Here's how the part is built. I have some questions about the finished solid (model axes, mm). Round coordinates to 2 decimals unless told otherwise and drop trailing zeros. Loops run counter-clockwise (first coordinate to the right, second up) from the corner with the lowest first, then second, coordinate; pieces in that order, holes last. Notation, with made-up numbers: (-18, -22.5) - (26, -22.5) arc R28 cw to (26, -2.5) - close; hole circle Ø4 at (12.5, 31.5). An arc over 180 degrees is marked (long way). Return JSON: item names as keys, results as strings. Group by question number.
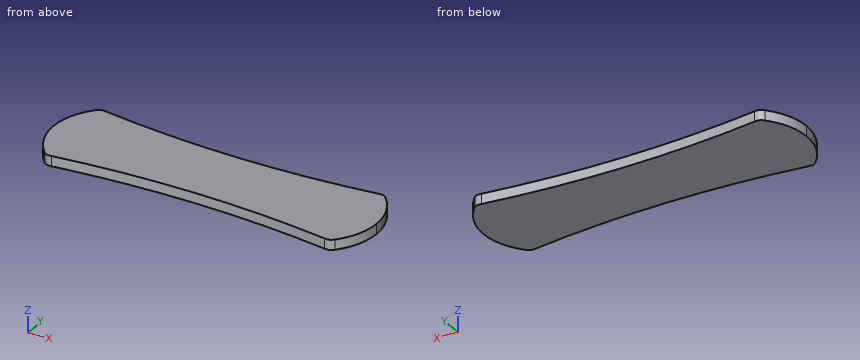
```python
from build123d import *

# Parameters (mm, degrees)
F1_DEPTH    = 25.4
F2_T1_DEPTH = 93.9988541888


# Not quite as in the source:
# - a fillet or chamfer that OpenCascade refuses, or shapes differently, is made with other operations: its cross-section is extruded or revolved along the edge and cut away or added


with BuildPart() as f1:
    # F0 (on Top) → F1 (new body)
    with BuildSketch(Plane.XY):
        with BuildLine():
            ThreePointArc((50.8, 558.8), (13.2719441568, 507.0402470414), (0, 444.5))
            ThreePointArc((0, 444.5), (13.2719441568, 381.9597529586), (50.8, 330.2))
            Line((50.8, 330.2), (50.8, 558.8))
        make_face()
        with BuildLine():
            ThreePointArc((277.2968022896, 536.7332159534), (163.7973759268, 545.1900472484), (50.8, 558.8))
            Line((50.8, 558.8), (50.8, 330.2))
            ThreePointArc((50.8, 330.2), (163.7973759268, 343.8099527516), (277.2968022896, 352.2667840466))
            ThreePointArc((277.2968022896, 352.2667840466), (300.1043048901, 395.8992851393), (307.975, 444.5))
            ThreePointArc((307.975, 444.5), (300.1043048901, 493.1007148607), (277.2968022896, 536.7332159534))
        make_face()
        with BuildLine():
            Line((762, 330.2), (762, 558.8))
            ThreePointArc((762, 558.8), (649.0026240732, 545.1900472484), (535.5031977104, 536.7332159534))
            ThreePointArc((535.5031977104, 536.7332159534), (504.825, 444.5), (535.5031977104, 352.2667840466))
            ThreePointArc((535.5031977104, 352.2667840466), (649.0026240732, 343.8099527516), (762, 330.2))
        make_face()
        with BuildLine():
            ThreePointArc((812.8, 444.5), (799.5280558432, 507.0402470414), (762, 558.8))
            Line((762, 558.8), (762, 330.2))
            ThreePointArc((762, 330.2), (799.5280558432, 381.9597529586), (812.8, 444.5))
        make_face()
        with BuildLine():
            ThreePointArc((535.5031977104, 536.7332159534), (406.4, 533.4), (277.2968022896, 536.7332159534))
            ThreePointArc((277.2968022896, 536.7332159534), (300.1043048901, 493.1007148607), (307.975, 444.5))
            ThreePointArc((307.975, 444.5), (300.1043048901, 395.8992851393), (277.2968022896, 352.2667840466))
            ThreePointArc((277.2968022896, 352.2667840466), (406.4, 355.6), (535.5031977104, 352.2667840466))
            ThreePointArc((535.5031977104, 352.2667840466), (504.825, 444.5), (535.5031977104, 536.7332159534))
        make_face()
    extrude(amount=F1_DEPTH)

    # F2: fillet of radius 25.4 on 4 edges, made by hand

    # F2_s2 → F2_t1 (cut)
    with BuildSketch(Plane.XY.offset(-34.2994270944)):
        with BuildLine():
            add(Edge.make_bspline(
                [(771.7640751065, 549.1617974106), (762.7642490879, 558.8744580913), (749.6481348223, 557.0578149138)],
                knots=[0, 0, 0, 1, 1, 1], degree=2, weights=[1, 1.5, 1]))
            ThreePointArc((749.6481348223, 557.0578149138), (755.8251531993, 557.9212093603), (762, 558.8))
            ThreePointArc((762, 558.8), (766.9894323112, 554.0896960119), (771.7640751065, 549.1617974106))
        make_face()
        with BuildLine():
            add(Edge.make_bspline(
                [(41.0359248935, 549.1617974105), (50.0357509121, 558.8744580913), (63.1518651777, 557.0578149137)],
                knots=[0, 0, 0, 1, 1, 1], degree=2, weights=[1, 1.5, 1]))
            ThreePointArc((63.1518651777, 557.0578149137), (56.9748468007, 557.9212093602), (50.8, 558.8))
            ThreePointArc((50.8, 558.8), (45.8105676888, 554.0896960119), (41.0359248935, 549.1617974105))
        make_face()
        with BuildLine():
            add(Edge.make_bspline(
                [(41.0359248935, 339.8382025894), (50.0357509121, 330.1255419087), (63.1518651777, 331.9421850862)],
                knots=[0, 0, 0, 1, 1, 1], degree=2, weights=[1, 1.5, 1]))
            ThreePointArc((63.1518651777, 331.9421850862), (56.9748468007, 331.0787906397), (50.8, 330.2))
            ThreePointArc((50.8, 330.2), (45.8105676888, 334.9103039881), (41.0359248935, 339.8382025894))
        make_face()
        with BuildLine():
            add(Edge.make_bspline(
                [(749.6481348223, 331.9421850862), (762.7642490879, 330.1255419087), (771.7640751065, 339.8382025894)],
                knots=[0, 0, 0, 1, 1, 1], degree=2, weights=[1, 1.5, 1]))
            ThreePointArc((771.7640751065, 339.8382025894), (766.9894323112, 334.9103039881), (762, 330.2))
            ThreePointArc((762, 330.2), (755.8251531993, 331.0787906397), (749.6481348223, 331.9421850862))
        make_face()
    extrude(amount=F2_T1_DEPTH, mode=Mode.SUBTRACT)


solid = f1.part
```
Q1. Please list where these lines run through material, in increasing order: line 1 (Y direction, x = 569, z = 20.25); line 2 (X direction, y = 360.5, z = 22); line 3 (X direction, y = 407.5, z = 20.5).
Q2. Imagine slicing it at B-B, the plane y = 400. List the corners of the cut face in (x, z) for me.
Q3. Imagine slicing it at A-A, the plane x = 651.5. List the corners of the cut face in (y, z) for me, and give its area (3 significant figures).
Q4. Will these pins go through, and if not, where does the flat tip stop? pin 1 Ø8 at (y, z) = (499.5, 22.5) entering from +X; pin 2 Ø8 at (y, z) = (371.5, 9) entering from +X; pin 3 Ø2 at (y, z) = (510.5, 17) entering from +X.
Output values:
{
 "1": {"line 1": "y = 350.31 to 538.69", "line 2": "x = 24.93 to 787.87", "line 3": "x = 4.51 to 808.29"},
 "2": {"outline": "(6.57, 0) - (806.23, 0) - (806.23, 25.4) - (6.57, 25.4) - close"},
 "3": {"outline": "(343.57, 0) - (545.43, 0) - (545.43, 25.4) - (343.57, 25.4) - close", "area": "5,130 mm^2"},
 "4": {"pin 1": "stops at x = 804.11", "pin 2": "stops at x = 796.48", "pin 3": "stops at x = 798.41"}
}
